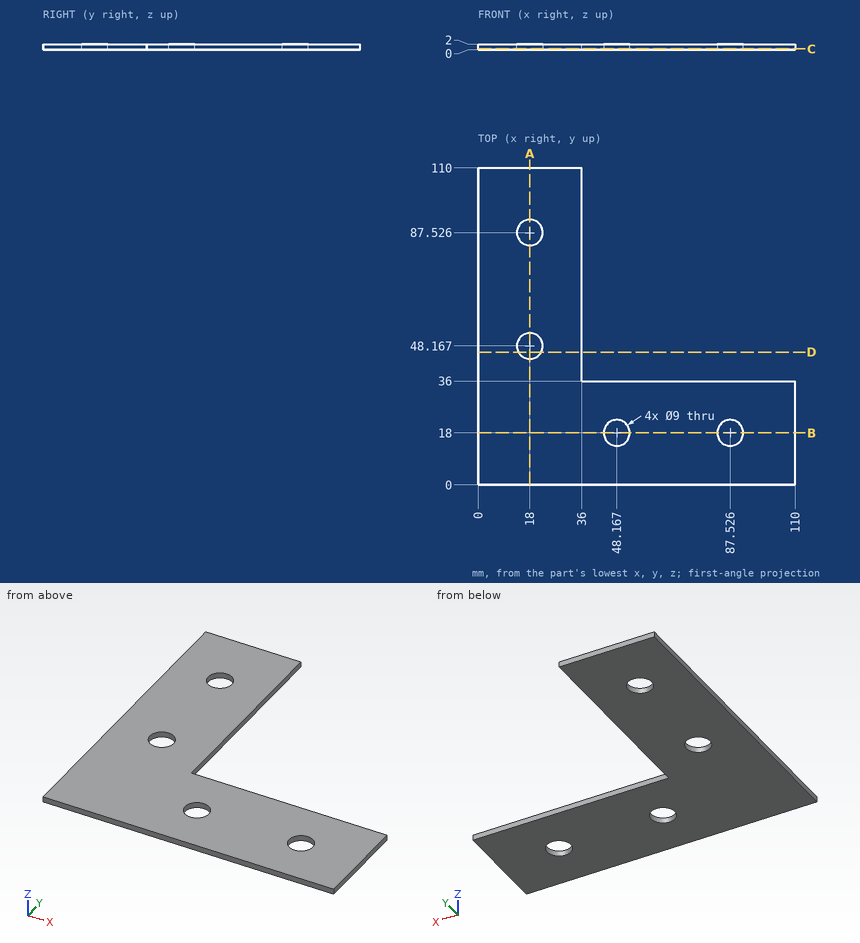
Geometry check sheet. Reference: drawing and pictorial views, mm from the part's lowest x, y, z. Round coordinates to 2 decimals unless told otherwise and drop trailing zeros. Order: outer loops, then holes, each group sorted by start corner. A loop starts at its lowest first (then second) coordinate and runs counter-clockwise, first axis right, second up.
Q1. Cross-section at A-A, the plane x = 18. Enter the section's corners in (y, z).
Filled sheet:
outline: (0, 0) - (43.67, 0) - (43.67, 2) - (0, 2) - close; (52.67, 0) - (83.03, 0) - (83.03, 2) - (52.67, 2) - close; (92.03, 0) - (110, 0) - (110, 2) - (92.03, 2) - close
Q2. Cross-section at C-C, the plane z = 0.3. Enter the section's corners in (x, y), plus the area to 3 significant figures.
Filled sheet:
outline: (0, 0) - (110, 0) - (110, 36) - (36, 36) - (36, 110) - (0, 110) - close; hole circle Ø9 at (18, 48.17); hole circle Ø9 at (18, 87.53); hole circle Ø9 at (48.17, 18); hole circle Ø9 at (87.53, 18)
area: 6,370 mm2
Q3. Scan lines: L1, parallel to Y at x = 18, z = 0.8; L2, parallel to Y at x = 70, z = 1.65. Record each from-to range of solid material in increasing order.
Filled sheet:
L1: y = 0 to 43.67, 52.67 to 83.03, 92.03 to 110
L2: y = 0 to 36
Q4. Cross-section at D-D, the plane y = 46. Enter the section's corners in (x, z).
Filled sheet:
outline: (0, 0) - (14.06, 0) - (14.06, 2) - (0, 2) - close; (21.94, 0) - (36, 0) - (36, 2) - (21.94, 2) - close
